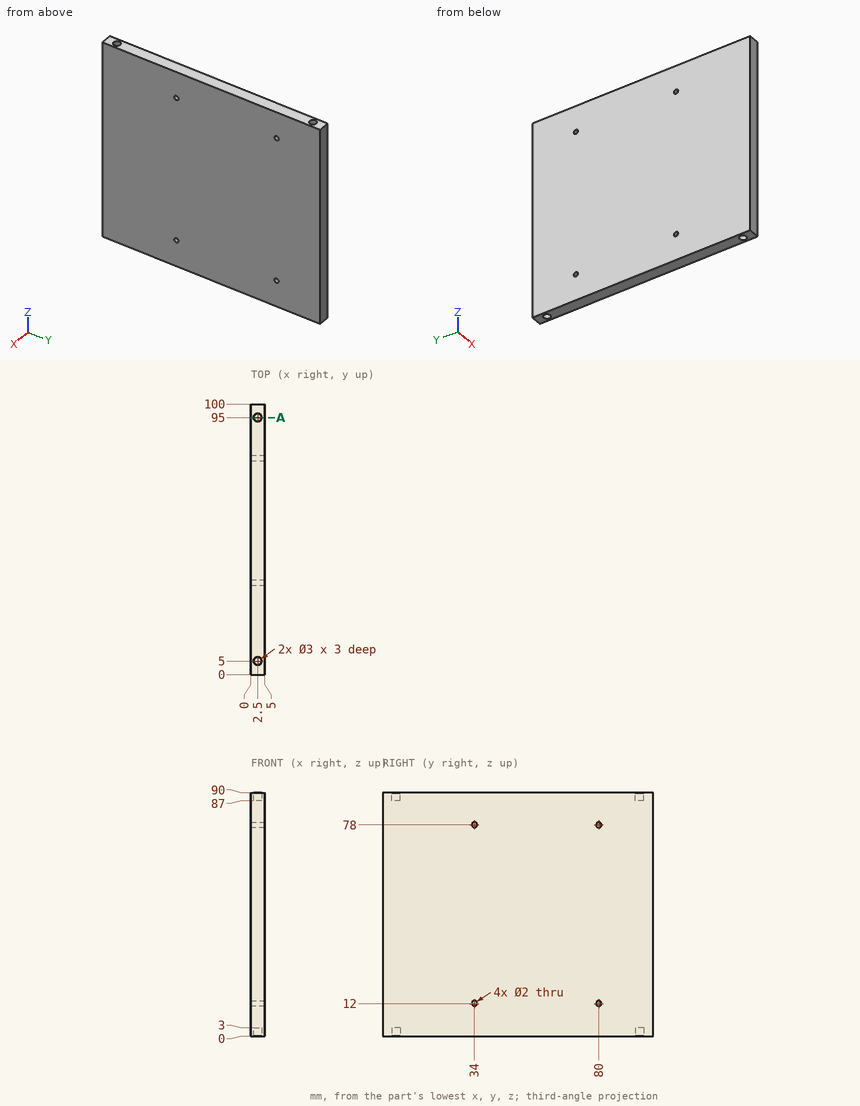
Geometry check sheet. Reference: drawing and pictorial views, mm from the part's lowest x, y, z. Give positions to 0.01 mm unless a question says otherwise; leave off trailing zeros. Order: outer loops, then holes, each group sorted by start corner. A loop starts at its lowest first (then second) coordinate and runs counter-clockwise, first axis right, second up. Notation, with made-up numbers: M 36,20.5 L 54,20.5 A31 ccw 54,59.5 Z; hole C 4.25,9.5 d11. An arc over 180 degrees is marked long. Answer in a Markdown table with one row per item. Add a question column.
Q1. Gauge pin test, flat ends, axial feed: pin 1 Ø0.9 at (x, y) = (2, 95) entering from -Z; pin 2 Ø1.2 at (y, z) = (34, 12) entering from +X; pin 3 Ø2.5 at (x, y) = (2.5, 5) entering from +Z. Record the tip position at first contact, or that the pin passes through.
Q2. Thickness scan on L1, parallel to Y at x = 2, z = 12; L2, parallel to Y at x = 2.5, z = 89.25; L3, parallel to Z at x = 3.75, y = 80. Record the ranges inside material, lowest first.
Q3. Sectioned sample at A-A, the plane y = 95. Record the boundary of the cut face in (x, z), and give its area (3 significant figures).
Verdict:
| question | item | result |
|---|---|---|
| 1 | pin 1 | z = 3 |
| 1 | pin 2 | through |
| 1 | pin 3 | z = 87 |
| 2 | L1 | 0 to 33, 35 to 79, 81 to 100 |
| 2 | L2 | 0 to 3.5, 6.5 to 93.5, 96.5 to 100 |
| 2 | L3 | 0 to 11, 13 to 77, 79 to 90 |
| 3 | outline | M 0,0 L 1,0 L 1,3 L 4,3 L 4,0 L 5,0 L 5,90 L 4,90 L 4,87 L 1,87 L 1,90 L 0,90 Z |
| 3 | area | 432 mm² |
